```python
from build123d import *

# Parameters (mm, degrees)
F0_W     = 14
F0_H     = 4.2391675711
F0_W_2   = 4
F0_H_2   = 28
F1_DEPTH = 2
F0_W_3   = 6
F0_H_3   = 2
F0_H_4   = 1.5
F2_DEPTH = 7
F3_R     = 1.74999
F4_R     = 1.25
F5_DEPTH = 25
F6_R     = 0.99999


# Not quite as in the source:
# - a fillet or chamfer is up to 0.001 mm smaller than in the source, because OpenCascade refuses the exact size
# - a feature names something its author has since deleted; it is built from what else it names


with BuildPart() as f1:
    # F0 (on Top) → F1 (new body)
    with BuildSketch(Plane.XY):
        with BuildLine():
            Line((-10, -26), (10, -26))
            ThreePointArc((10, -26), (12.9289321881, -18.9289321881), (20, -16))
            Line((20, -16), (20, 16))
            ThreePointArc((20, 16), (12.9289321881, 18.9289321881), (10, 26))
            Line((10, 26), (-10, 26))
            ThreePointArc((-10, 26), (-12.9289321881, 18.9289321881), (-20, 16))
            Line((-20, 16), (-20, -16))
            ThreePointArc((-20, -16), (-12.9289321881, -18.9289321881), (-10, -26))
        make_face()
        with Locations((0, -22.1195837855)):
            Rectangle(F0_W, F0_H, mode=Mode.SUBTRACT)
        with Locations((-16, 0)):
            Rectangle(F0_W_2, F0_H_2, mode=Mode.SUBTRACT)
        Polygon((3, 18), (10, 18), (12, 18), (12, -18), (-12, -18), (-12, 18), (-10, 18), (-3, 18), (-3, 19.5), (3, 19.5), align=None, mode=Mode.SUBTRACT)
        with Locations((16, 0)):
            Rectangle(F0_W_2, F0_H_2, mode=Mode.SUBTRACT)
        with Locations((0, 22.1195837855)):
            Rectangle(F0_W, F0_H, mode=Mode.SUBTRACT)
        with BuildLine():
            Line((-20, 24.75), (-20, 16))
            ThreePointArc((-20, 16), (-12.9289321881, 18.9289321881), (-10, 26))
            Line((-10, 26), (-18.75, 26))
            ThreePointArc((-18.75, 26), (-19.1161165235, 25.1161165235), (-20, 24.75))
        make_face()
        with BuildLine():
            Line((-25.7454968465, 22.5147810633), (-20, 16))
            Line((-20, 16), (-20, 24.75))
            ThreePointArc((-20, 24.75), (-20.8838834765, 26.8838834765), (-18.75, 26))
            Line((-18.75, 26), (-10, 26))
            Line((-10, 26), (-21.386597903, 31.5147810633))
            Line((-21.386597903, 31.5147810633), (-25.7454968465, 22.5147810633))
        make_face()
        with BuildLine():
            ThreePointArc((10, 26), (12.9289321881, 18.9289321881), (20, 16))
            Line((20, 16), (20, 24.75))
            ThreePointArc((20, 24.75), (19.1161165235, 25.1161165235), (18.75, 26))
            Line((18.75, 26), (10, 26))
        make_face()
        with BuildLine():
            Line((20, 24.75), (20, 16))
            Line((20, 16), (25.7454968465, 22.5147810633))
            Line((25.7454968465, 22.5147810633), (21.386597903, 31.5147810633))
            Line((21.386597903, 31.5147810633), (10, 26))
            Line((10, 26), (18.75, 26))
            ThreePointArc((18.75, 26), (20, 27.25), (21.25, 26))
            ThreePointArc((21.25, 26), (20.8838834765, 25.1161165235), (20, 24.75))
        make_face()
        with BuildLine():
            ThreePointArc((20, -16), (12.9289321881, -18.9289321881), (10, -26))
            Line((10, -26), (18.75, -26))
            ThreePointArc((18.75, -26), (19.1161165235, -25.1161165235), (20, -24.75))
            Line((20, -24.75), (20, -16))
        make_face()
        with BuildLine():
            Line((18.75, -26), (10, -26))
            Line((10, -26), (21.386597903, -31.5147810633))
            Line((21.386597903, -31.5147810633), (25.7454968465, -22.5147810633))
            Line((25.7454968465, -22.5147810633), (20, -16))
            Line((20, -16), (20, -24.75))
            ThreePointArc((20, -24.75), (20.8838834765, -25.1161165235), (21.25, -26))
            ThreePointArc((21.25, -26), (20, -27.25), (18.75, -26))
        make_face()
        with BuildLine():
            Line((-21.386597903, -31.5147810633), (-10, -26))
            Line((-10, -26), (-18.75, -26))
            ThreePointArc((-18.75, -26), (-20.8838834765, -26.8838834765), (-20, -24.75))
            Line((-20, -24.75), (-20, -16))
            Line((-20, -16), (-25.7454968465, -22.5147810633))
            Line((-25.7454968465, -22.5147810633), (-21.386597903, -31.5147810633))
        make_face()
        with BuildLine():
            Line((-18.75, -26), (-10, -26))
            ThreePointArc((-10, -26), (-12.9289321881, -18.9289321881), (-20, -16))
            Line((-20, -16), (-20, -24.75))
            ThreePointArc((-20, -24.75), (-19.1161165235, -25.1161165235), (-18.75, -26))
        make_face()
    extrude(amount=F1_DEPTH)

    # F0 (on Top) → F2 (join)
    with BuildSketch(Plane.XY):
        with Locations((0, 17)):
            Rectangle(F0_W_3, F0_H_3)
        with Locations((0, 18.75)):
            Rectangle(F0_W_3, F0_H_4)
    extrude(amount=F2_DEPTH)

    # F3 (radius 1.75 in the source; OpenCascade refuses exactly that, so slightly less here)
    f3_edges = [f1.edges().sort_by_distance(p)[0] for p in [
        (0, 16, 7),
        (0, 19.5, 7),
    ]]
    fillet(f3_edges, radius=F3_R)

    # F4 (on face) → F5 (cut)
    with BuildSketch(Plane(origin=(-3, 0, 0), x_dir=(0, -1, 0), z_dir=(-1, 0, 0))):
        with Locations((-17.75, 5)):
            Circle(F4_R)
    extrude(amount=-F5_DEPTH, mode=Mode.SUBTRACT)

    # F6 (radius 1 in the source; OpenCascade refuses exactly that, so slightly less here)
    f6_edges = [f1.edges().sort_by_distance(p)[0] for p in [
        (-20, 0, 2),
        (-23.566047, -27.014781, 2),
        (0, -26, 2),
        (20, 0, 2),
        (15.693299, 28.757391, 2),
        (0, 26, 2),
        (-23.566047, 27.014781, 2),
        (-23.566047, 27.014781, 0),
        (0, 26, 0),
        (15.693299, 28.757391, 0),
        (20, 0, 0),
        (-23.566047, -27.014781, 0),
        (0, -26, 0),
        (-20, 0, 0),
        (-12, 0, 2),
        (-7.5, 18, 2),
        (7.5, 18, 2),
        (12, 0, 2),
        (0, -18, 2),
        (0, 16, 0),
        (-12, 0, 0),
        (0, -18, 0),
        (12, 0, 0),
        (-22.872748, 19.257391, 2),
        (-22.872748, 19.257391, 0),
        (-15.693299, 28.757391, 2),
        (-15.693299, 28.757391, 0),
        (22.872748, 19.257391, 2),
        (22.872748, 19.257391, 0),
        (22.872748, -19.257391, 2),
        (22.872748, -19.257391, 0),
        (15.693299, -28.757391, 0),
        (15.693299, -28.757391, 2),
        (-15.693299, -28.757391, 0),
        (-15.693299, -28.757391, 2),
        (-22.872748, -19.257391, 0),
        (-22.872748, -19.257391, 2),
        (7.5, 18, 0),
        (-7.5, 18, 0),
        (23.566047, -27.014781, 2),
        (23.566047, -27.014781, 0),
        (23.566047, 27.014781, 2),
        (23.566047, 27.014781, 0),
    ]]
    fillet(f6_edges, radius=F6_R)


solid = f1.part
```
Input: part model. Units: mm. Frame: model coordinates. A direction names the side the tool comes from. Round coordinates to 2 decimals unless told otherwise and drop trailing zeros. One line per item, written item: value.
(1) Set-up query: faces 1 (the face through (-14, 0, 1)), 2 (the face through (-15.64, -28.4, 0.29)), 3 (the face through (15.64, 28.4, 1.71)), 4 (the face through (22.48, -19.267, 0.285)). Return all of +Z, -Z, +X, -X, +Y, -Y with unobstructed straight access to the full face (end or side cutting, diameter ignored); none if empty.
Geometry check:
face 1: +Z, -Z
face 2: -Z, -Y
face 3: +Z, +Y
face 4: -Z, +X
(2) Section A-A (y = 13). Give the number of separate pieces and of enclosed holes in the cut face, plus the area to 3 significant figures.
Geometry check:
separate pieces: 4
enclosed holes: 0
area: 14.3 mm2
(3) Material intervals for line 1 (X direction, y = -26, z = 0.4); line 2 (X direction, y = 26, z = 0.6); line 3 (Y direction, x = 9.5, z = 1), sorted ascending. Write a range as [from, to].
Geometry check:
line 1: [-23.84, -21.25], [-18.75, -10.46], [10.46, 18.75], [21.25, 23.84]
line 2: [-23.96, -21.25], [-18.75, -10.19], [10.19, 18.75], [21.25, 23.96]
line 3: [-26, -18], [18, 26]
(4) Mould query, pull axis X, two halves, no side actions, for faces 5 (the face through (-22.48, 19.267, 1.715)), 6 (the face through (22.48, -19.267, 1.715)), 7 (the face through (-7, -22, 1)). Classes: pulls with the +X half, pulls with the -X half, needs draft (parallel to the pull), parting line crosses it, or undercut.
Geometry check:
face 5: pulls with the -X half
face 6: pulls with the +X half
face 7: undercut
(5) Pin query (flat end, axial travel): pin 1 (0.6 mm diameter, centred on x = 16.5, z = 1, fed in from +Y); pin 2 (2 mm diameter, centred on x = 16, z = 1, fed in from -Y); pin 3 (4 mm diameter, centred on x = -2, z = 6, fed in from -Y). Return the tip coordinate at first contact, or that it passes through.
Geometry check:
pin 1: y = 29.29
pin 2: y = -29.39
pin 3: y = 16
